Geometry check sheet. Reference: the model listing, model coordinates, mm. Face numbers are marked on the shaded views. Round coordinates to 2 decimals unless told otherwise and drop trailing zeros. Order: outer loops, then holes, each group sorted by start corner. A loop starts at its lowest first (then second) coordinate and runs counter-clockwise, first axis right, second up.
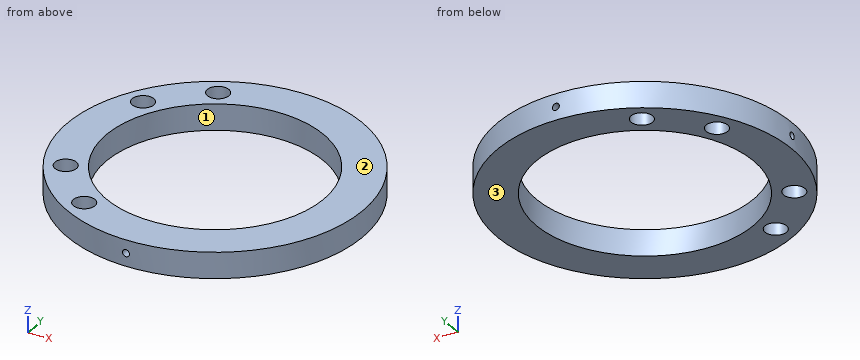
```python
from build123d import *

# Parameters (mm, degrees)
SKETCH_R              = 42.45
SKETCH_R_2            = 31.25
PAD_DEPTH             = 7.5
SKETCH011_R           = 3.1
POCKET003_DEPTH       = 7.501
SKETCH024_R           = 1
POCKET012_DEPTH       = 6
POLARPATTERN001_COUNT = 3
POLARPATTERN001_ANGLE = 180


with BuildPart() as part:
    # Sketch → Pad (new body)
    with BuildSketch(Plane.XY):
        Circle(SKETCH_R)
        Circle(SKETCH_R_2, mode=Mode.SUBTRACT)
    extrude(amount=PAD_DEPTH)

    # Sketch011 (on DatumPlane) → Pocket003 (cut, through all)
    with BuildSketch(Plane.XY.offset(7.5)):
        with Locations((-31.913036, 18.425)):
            Circle(SKETCH011_R)
        with Locations((-31.913036, -18.425)):
            Circle(SKETCH011_R)
        with Locations((-18.425, 31.913036)):
            Circle(SKETCH011_R)
        with Locations((-18.425, -31.913036)):
            Circle(SKETCH011_R)
    extrude(amount=-POCKET003_DEPTH, mode=Mode.SUBTRACT)

    # Sketch024 (on DatumPlane) → Pocket012 (cut)
    with BuildSketch(Plane.XZ.offset(42.45)):
        with Locations((0, 3.75)):
            Circle(SKETCH024_R)
    pocket012 = extrude(amount=-POCKET012_DEPTH, mode=Mode.SUBTRACT)

    # PolarPattern001: Pocket012 ×3 about axis
    polarpattern001_axis = Axis((0, 0, 0), (0, 0, -1))
    for i in range(1, POLARPATTERN001_COUNT):
        add(pocket012.rotate(polarpattern001_axis, i * POLARPATTERN001_ANGLE / (POLARPATTERN001_COUNT - 1)), mode=Mode.SUBTRACT)


with BuildPart() as part_1:
    # Body placement: moved
    add(part.part.moved(Location((0, 0, -12))))


solid = part_1.part
```
(1) Sectioned sample at A-A, the plane y = 0. Record the cut outline in (x, z), and give its area (3 significant figures).
Returned:
outline: (-42.45, -12) - (-31.25, -12) - (-31.25, -4.5) - (-42.45, -4.5) - (-42.45, -7.25) - (-36.45, -7.25) - (-36.45, -9.25) - (-42.45, -9.25) - close; (31.25, -12) - (42.45, -12) - (42.45, -4.5) - (31.25, -4.5) - close
area: 156 mm2
(2) Depth check by flat-ended pin: P1, Ø5, axis at x = -31.91, y = 18.42, coming from the +Z side; P2, Ø1, axis at y = -18, z = -10, coming from the -X side; P3, Ø1, axis at x = 0, z = -8, coming from the +Y side; P4, Ø0.6, axis at y = -0.5, z = -8, coming from the -X side. Enter the tip coordinate at first touch or a pass-through.
Returned:
P1: passes through
P2: stops at x = -38.67
P3: stops at y = 36.45
P4: stops at x = -36.45
(3) Material ranges on line 1 (Y direction, x = -1, z = -10.5); line 2 (Z direction, x = 0, y = -39.5); line 3 (X direction, y = -16.5, z = -6), recorded low to high.
Returned:
line 1: y = -42.44 to -31.23, 31.23 to 42.44
line 2: z = -12 to -9.25, -7.25 to -4.5
line 3: x = -39.11 to -34.34, -29.48 to -26.54, 26.54 to 39.11
(4) Sectioned sample at D-D, the plane y = 17. Record the cut outline in (x, z).
Returned:
outline: (-38.9, -12) - (-34.67, -12) - (-34.67, -4.5) - (-38.9, -4.5) - close; (-29.16, -12) - (-26.22, -12) - (-26.22, -4.5) - (-29.16, -4.5) - close; (26.22, -12) - (38.9, -12) - (38.9, -4.5) - (26.22, -4.5) - close
(5) Draft check along Z on the marked faces 1, 2 and 3. Enter one of: released by +Z, released by -Z, zero draft, split by the parting line, or undercut.
Returned:
face 1: zero draft
face 2: released by +Z
face 3: released by -Z
(6) Sectioned sample at C-C, the plane z = -8.25. Record the cut outline in (x, y) (3 decimals).
Returned:
outline: (-42.438, -1) arc R42.45 ccw to (-1, -42.438) - (-1, -36.45) - (1, -36.45) - (1, -42.438) arc R42.45 ccw to (1, 42.438) - (1, 36.45) - (-1, 36.45) - (-1, 42.438) arc R42.45 ccw to (-42.438, 1) - (-36.45, 1) - (-36.45, -1) - close; hole circle Ø6.2 at (-31.913, -18.425); hole circle Ø6.2 at (-31.913, 18.425); hole circle Ø62.5 at (0, 0); hole circle Ø6.2 at (-18.425, -31.913); hole circle Ø6.2 at (-18.425, 31.913)
(7) Sectioned sample at B-B, the plane x = 0. Record the cut outline in (y, z).
Returned:
outline: (-42.45, -12) - (-31.25, -12) - (-31.25, -4.5) - (-42.45, -4.5) - (-42.45, -7.25) - (-36.45, -7.25) - (-36.45, -9.25) - (-42.45, -9.25) - close; (31.25, -12) - (42.45, -12) - (42.45, -9.25) - (36.45, -9.25) - (36.45, -7.25) - (42.45, -7.25) - (42.45, -4.5) - (31.25, -4.5) - close
